Geometry check sheet. Reference: the model listing, model coordinates, mm. Face numbers are marked on the shaded views. Give positions to 0.01 mm unless a question says otherwise; leave off trailing zeros. Loops run counter-clockwise (first coordinate to the right, second up) from the corner with the lowest first, then second, coordinate; pieces in that order, holes last. Notation, with made-up numbers: (77.25, 80) -> (95.25, 80) arc R23 cw to (95.25, 108) -> close; hole circle Ø4 at (49, -6.5). An arc over 180 degrees is marked (long way). One line per item, written item: value. Start each with the question number.
(1) Gauge pin test, flat ends, axial feed: pin 1 Ø12 at (x, y) = (-13, 8) entering from +Z; pin 2 Ø12 at (x, z) = (7.5, -11.5) entering from +Y; pin 3 Ø3 at (x, y) = (-2.5, 33) entering from +Z. Record the tip position at first contact, or that the pin passes through.
(2) Scan lines: line 1 along X through (y, z) = (5.75, 0); line 2 along Y through (x, z) = (-2, -10). Record each from-to range of solid material in increasing order. Write a range as from..to.
(3) Draft check along Y on the marked faces 1, 2 and 3. Enter one of: pulls with the +Y half, pulls with the -Y half, needs draft (parallel to the pull), parting line crosses it, or undercut.
(4) Sectioned sample at B-B, the plane x = 0. Record the cut outline in (y, z).
(5) Sectioned sample at C-C, the plane y = 5.5. Record the cut outline in (x, z).
(6) Sectioned sample at D-D, the plane y = 46. Record the cut outline in (x, z).
(7) Sectioned sample at A-A, the plane z = 0. Record the cut outline in (x, y), then the cut area to 3 significant figures.
from build123d import *

# Parameters (mm, degrees)
SKETCH1_R                = 21.166666667
SKETCH1_R_2              = 2.5
BOSS_EXTRUDE1_DEPTH      = 40
SKETCH2_R                = 2.5
BOSS_EXTRUDE2_DEPTH      = 10
BOSS_EXTRUDE2_DEPTH_BACK = 30


with BuildPart() as part:
    # Sketch1 → Boss-Extrude1 (new body)
    with BuildSketch(Plane(origin=(0, 0, 0), x_dir=(1, 0, 0), z_dir=(0, 1, 0))):
        Circle(SKETCH1_R)
        Circle(SKETCH1_R_2, mode=Mode.SUBTRACT)
    extrude(amount=BOSS_EXTRUDE1_DEPTH)

    # Sketch2 → Boss-Extrude2 (add, two sides)
    with BuildSketch(Plane(origin=(0, 40, 0), x_dir=(1, 0, 0), z_dir=(0, 1, 0))) as boss_extrude2_sk:
        Circle(SKETCH2_R)
    extrude(amount=BOSS_EXTRUDE2_DEPTH)
    extrude(boss_extrude2_sk.sketch, amount=-BOSS_EXTRUDE2_DEPTH_BACK)


solid = part.part
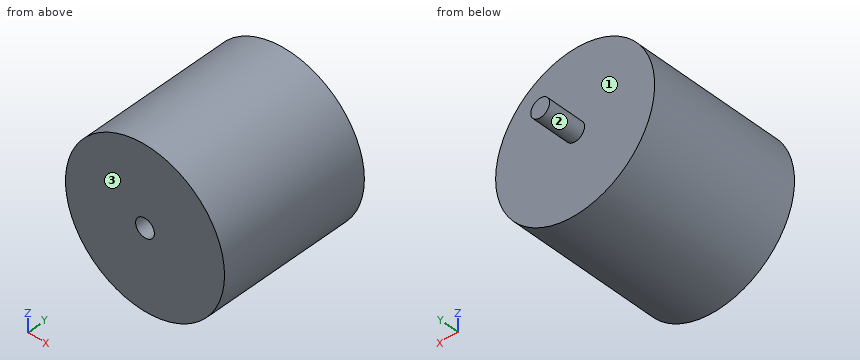
Calculated:
1. pin 1: stops at z = 19.98
1. pin 2: stops at y = 40
1. pin 3: stops at z = 21.14
2. line 1: x = -21.17..-2.5, 2.5..21.17
2. line 2: y = 0..40
3. face 1: pulls with the +Y half
3. face 2: needs draft
3. face 3: pulls with the -Y half
4. outline: (0, -21.17) -> (40, -21.17) -> (40, -2.5) -> (50, -2.5) -> (50, 2.5) -> (40, 2.5) -> (40, 21.17) -> (0, 21.17) -> (0, 2.5) -> (10, 2.5) -> (10, -2.5) -> (0, -2.5) -> close
5. outline: circle Ø42.33 at (0, 0); hole circle Ø5 at (0, 0)
6. outline: circle Ø5 at (0, 0)
7. outline: (-21.17, 0) -> (-2.5, 0) -> (-2.5, 10) -> (2.5, 10) -> (2.5, 0) -> (21.17, 0) -> (21.17, 40) -> (2.5, 40) -> (2.5, 50) -> (-2.5, 50) -> (-2.5, 40) -> (-21.17, 40) -> close
7. area: 1,690 mm2
